Verification items for the finished model (mm, model axes). Face numbers are marked on the shaded views. Give positions to 0.01 mm unless a question says otherwise; leave off trailing zeros. Order: outer loops, then holes, each group sorted by start corner. A loop starts at its lowest first (then second) coordinate and runs counter-clockwise, first axis right, second up.
from build123d import *

# Parameters (mm, degrees)
SKETCH_1_R               = 15.2
EXTRUDE_2_DEPTH          = 5
CUT_EXTRUDE_1_DEPTH      = 23.069888989
CUT_EXTRUDE_1_DEPTH_BACK = 23.069888989
SKETCH_3_R               = 1.25
CUT_EXTRUDE_2_DEPTH      = 23.069888989
CUT_EXTRUDE_2_DEPTH_BACK = 23.069888989
SKETCH_4_R               = 2


with BuildPart() as part:
    # 草图1 → 凸台-拉伸2 (new body)
    with BuildSketch(Plane.XY):
        Circle(SKETCH_1_R)
    extrude(amount=EXTRUDE_2_DEPTH)

    # 草图3 → 切除-拉伸1 (cut, two sides: drawn at the far end of the back side and taken through both)
    with BuildSketch(Plane.XY.offset(5).offset(-CUT_EXTRUDE_1_DEPTH_BACK)):
        with Locations((0, 12.5)):
            Circle(SKETCH_3_R)
        with Locations((10.825317547, 6.25)):
            Circle(SKETCH_3_R)
        with Locations((10.825317547, -6.25)):
            Circle(SKETCH_3_R)
        with Locations((0, -12.5)):
            Circle(SKETCH_3_R)
        with Locations((-10.825317547, -6.25)):
            Circle(SKETCH_3_R)
        with Locations((-10.825317547, 6.25)):
            Circle(SKETCH_3_R)
    extrude(amount=CUT_EXTRUDE_1_DEPTH + CUT_EXTRUDE_1_DEPTH_BACK, mode=Mode.SUBTRACT)

    # 草图4 → 切除-拉伸2 (cut, two sides: drawn at the far end of the back side and taken through both)
    with BuildSketch(Plane.XY.offset(5).offset(-CUT_EXTRUDE_2_DEPTH_BACK)):
        Circle(SKETCH_4_R)
    extrude(amount=CUT_EXTRUDE_2_DEPTH + CUT_EXTRUDE_2_DEPTH_BACK, mode=Mode.SUBTRACT)


solid = part.part
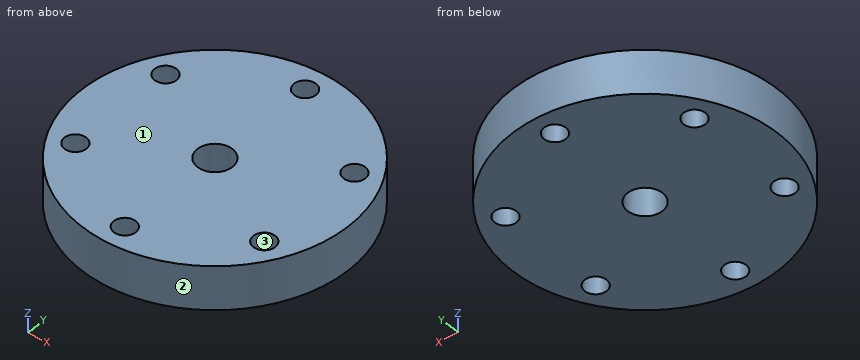
(1) Scan lines: line 1 (Y direction, x = 0, z = 1.55); line 2 (Y direction, x = -11.5, z = 1); line 3 (X direction, y = 6.25, z = 1). Record each from-to range of solid material in increasing order.
Solved:
line 1: y = -15.2 to -13.75, -11.25 to -2, 2 to 11.25, 13.75 to 15.2
line 2: y = -9.94 to -7.3, -5.2 to 5.2, 7.3 to 9.94
line 3: x = -13.86 to -12.08, -9.58 to 9.58, 12.08 to 13.86
(2) Release check for a two-part mould opening along X. For the marked faces 1, 2 and 3 record: pulls with the +X half, pulls with the -X half, needs draft (parallel to the pull), parting line crosses it, or undercut.
Solved:
face 1: needs draft
face 2: parting line crosses it
face 3: undercut
(3) Go/stop test with flat-tipped pins: pin 1 (2.5 mm diameter, centred on x = 0, y = 0, fed in from -Z); pin 2 (2 mm diameter, centred on x = 5.5, z = 2.5, fed in from +Y); pin 3 (2 mm diameter, centred on y = 7, z = 2.5, fed in from -X). Record where each tip stops, or that it passes through.
Solved:
pin 1: passes through
pin 2: stops at y = 14.52
pin 3: stops at x = -13.97
(4) Section check B-B, the plane y = 0. Enter the section's corners in (x, z), then the cut area to 3 significant figures.
Solved:
outline: (-15.2, 0) - (-2, 0) - (-2, 5) - (-15.2, 5) - close; (2, 0) - (15.2, 0) - (15.2, 5) - (2, 5) - close
area: 132 mm2
(5) Section check A-A, the plane x = 0. Enter the section's corners in (y, z), then the cut area to 3 significant figures.
Solved:
outline: (-15.2, 0) - (-13.75, 0) - (-13.75, 5) - (-15.2, 5) - close; (-11.25, 0) - (-2, 0) - (-2, 5) - (-11.25, 5) - close; (2, 0) - (11.25, 0) - (11.25, 5) - (2, 5) - close; (13.75, 0) - (15.2, 0) - (15.2, 5) - (13.75, 5) - close
area: 107 mm2
(6) Section check D-D, the plane y = 12.5. Enter the section's corners in (x, z), then the cut area to 3 significant figures.
Solved:
outline: (-8.65, 0) - (-1.25, 0) - (-1.25, 5) - (-8.65, 5) - close; (1.25, 0) - (8.65, 0) - (8.65, 5) - (1.25, 5) - close
area: 74.0 mm2
(7) Section check C-C, the plane y = 6.25. Enter the section's corners in (x, z), then the cut area to 3 significant figures.
Solved:
outline: (-13.86, 0) - (-12.08, 0) - (-12.08, 5) - (-13.86, 5) - close; (-9.58, 0) - (9.58, 0) - (9.58, 5) - (-9.58, 5) - close; (12.08, 0) - (13.86, 0) - (13.86, 5) - (12.08, 5) - close
area: 114 mm2
